Can you work these out from the model? Positions are in its coordinate system, mm. Round coordinates to 2 decimals unless told otherwise and drop trailing zeros. Loops run counter-clockwise (first coordinate to the right, second up) from the corner with the lowest first, then second, coordinate; pieces in that order, holes last. Notation, with made-up numbers: M 58,39.5 L 74,39.5 A35 ccw 74,73.5 Z; hole C 27.25,50 d8. An arc over 180 degrees is marked long. Return JSON: item names as keys, results as strings.
```python
from build123d import *

# Parameters (mm, degrees)
SKETCH_1_W          = 40
SKETCH_1_H          = 15
SKETCH_1_R          = 1
EXTRUDE_1_DEPTH     = 1.5
SKETCH_2_W          = 19.349402369
SKETCH_2_H          = 7.733193781
CUT_EXTRUDE_1_DEPTH = 1.5
FILLET_2_R          = 1
FILLET_3_R          = 2
EXTRUDE_2_DEPTH     = 1.5
FILLET_4_R          = 2


with BuildPart() as part:
    # 草图1 → 凸台-拉伸1 (new body)
    with BuildSketch(Plane.XY):
        with Locations((-3.988440653, 4.336799691)):
            Rectangle(SKETCH_1_W, SKETCH_1_H)
        with Locations((-21.738440653, 4.336799691)):
            Circle(SKETCH_1_R, mode=Mode.SUBTRACT)
        with Locations((13.761559347, 4.336799691)):
            Circle(SKETCH_1_R, mode=Mode.SUBTRACT)
    extrude(amount=EXTRUDE_1_DEPTH)

    # 草图2 → 切除-拉伸1 (cut)
    with BuildSketch(Plane.XY.offset(1.5)):
        with Locations((-7.602725981, 2.54307272)):
            Rectangle(SKETCH_2_W, SKETCH_2_H)
    extrude(amount=-CUT_EXTRUDE_1_DEPTH, mode=Mode.SUBTRACT)

    # 圆角2
    fillet_2_edges = [part.edges().sort_by_distance(p)[0] for p in [
        (16.011559347, -3.163200309, 0.75),
        (-23.988440653, -3.163200309, 0.75),
        (-23.988440653, 11.836799691, 0.75),
        (16.011559347, 11.836799691, 0.75),
    ]]
    fillet(fillet_2_edges, radius=FILLET_2_R)

    # 圆角3
    fillet_3_edges = [part.edges().sort_by_distance(p)[0] for p in [
        (2.071975204, 6.40966961, 0.75),
        (2.071975204, -1.323524171, 0.75),
        (-17.277427165, -1.323524171, 0.75),
        (-17.277427165, 6.40966961, 0.75),
    ]]
    fillet(fillet_3_edges, radius=FILLET_3_R)

    # 草图3 → 凸台-拉伸2 (add)
    with BuildSketch(Plane.XY.offset(1.5)):
        Polygon((-18.839640509, -2.587666371), (-16.040814973, -5.386491907), (-0.864084954, -5.386491907), (2.88813454, -1.634272413), align=None)
    extrude(amount=-EXTRUDE_2_DEPTH)

    # 圆角4
    fillet_4_edges = [part.edges().sort_by_distance(p)[0] for p in [
        (-18.26410657, -3.163200309, 0.75),
        (1.359206644, -3.163200309, 0.75),
        (-16.040814973, -5.386491907, 0.75),
        (-0.864084954, -5.386491907, 0.75),
    ]]
    fillet(fillet_4_edges, radius=FILLET_4_R)


solid = part.part
```
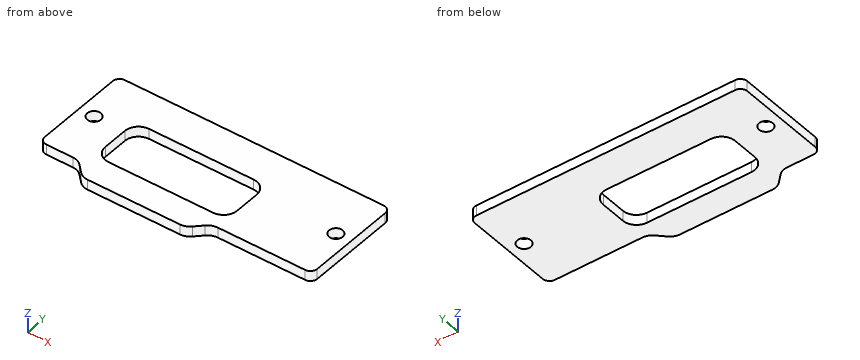
Q1. I'm going to push flat-ended pins straight in: pin 1 Ø1.6 at (x, y) = (13.76, 4.34) entering from -Z; pin 2 Ø2.5 at (x, y) = (-21.74, 4.34) entering from -Z. Where does each tip first touch, or does it pass through?
Results:
{"pin 1": "passes through", "pin 2": "stops at z = 0"}
Q2. If I drill on line 1 along X through (y, z) = (4.25, 0.5); line 2 along Y through (x, z) = (-7.5, 1.3); line 3 along Y through (x, z) = (12.5, 0.65), over which ranges is the centre line in solid material (lowest first)?
Results:
{"line 1": "x = -23.99 to -22.73, -20.74 to -17.28, 2.07 to 12.77, 14.76 to 16.01", "line 2": "y = -5.39 to -1.32, 6.41 to 11.84", "line 3": "y = -3.16 to 11.84"}
Q3. Suppose I cut it at A-A, the plane x = -14. Please give me the cut outline in (y, z), plus the area to 3 significant figures.
Results:
{"outline": "M -5.39,0 L -1.32,0 L -1.32,1.5 L -5.39,1.5 Z; M 6.41,0 L 11.84,0 L 11.84,1.5 L 6.41,1.5 Z", "area": "14.2 mm2"}
Q4. Suppose I cut it at C-C, the plane z = 0.5. Please give me the cut outline in (x, y).
Results:
{"outline": "M -23.99,-2.16 A1 ccw -22.99,-3.16 L -19.09,-3.16 A2 cw -17.68,-3.75 L -16.63,-4.8 A2 ccw -15.21,-5.39 L -1.69,-5.39 A2 ccw -0.28,-4.8 L 0.77,-3.75 A2 cw 2.19,-3.16 L 15.01,-3.16 A1 ccw 16.01,-2.16 L 16.01,10.84 A1 ccw 15.01,11.84 L -22.99,11.84 A1 ccw -23.99,10.84 Z; hole C -21.74,4.34 d2; hole M -17.28,0.68 A2 ccw -15.28,-1.32 L 0.07,-1.32 A2 ccw 2.07,0.68 L 2.07,4.41 A2 ccw 0.07,6.41 L -15.28,6.41 A2 ccw -17.28,4.41 Z; hole C 13.76,4.34 d2"}
Q5. Suppose I cut it at D-D, the plane x = -19.5. Please give me the cut outline in (y, z).
Results:
{"outline": "M -3.16,0 L 11.84,0 L 11.84,1.5 L -3.16,1.5 Z"}
Q6. Suppose I cut it at B-B, the plane y = 1.25. Please give me the cut outline in (x, z), plus the area to 3 significant figures.
Results:
{"outline": "M -23.99,0 L -17.28,0 L -17.28,1.5 L -23.99,1.5 Z; M 2.07,0 L 16.01,0 L 16.01,1.5 L 2.07,1.5 Z", "area": "31.0 mm2"}
